The model under review builds one solid part; all positions refer to its coordinate system, in mm. A direction names the side the tool comes from. Coordinates: 2 decimals unless noted, no trailing zeros. Order: outer loops, then holes, each group sorted by start corner. A loop starts at its lowest first (then second) coordinate and runs counter-clockwise, first axis right, second up. Notation, with made-up numbers: M 64,45.25 L 112,45.25 A15 ccw 112,59.25 Z; hole C 59,42.5 d11. An arc over 180 degrees is marked long. Answer as CSV lines item,"result". Start each with the question number.
Q1. Consider section A-A on x = 10. Write out the cut boundary in (y, z), and give its area (4 significant figures).
Q2. Consider section D-D on y = 16. Write out the cut boundary in (x, z).
Q3. The part is to be moulded in two halves that separate along Y. For faces 4 (the face through (10, 15, 6.25)), 5 (the face through (0, 17.5, 5)), say which applies: +Y half, -Y half, draft (parallel to the pull), parting line (faces both ways), or undercut.
Q4. Consider section C-C on z = 1.75. Write out the cut boundary in (x, y).
Q5. Consider section B-B on z = 5.25. Write out the cut boundary in (x, y).
Q6. Machinability: for faces 1 (the face through (-10, 15, 6.25)), 2 (the face through (5, 15, 3)), 3 (the face through (0, 22.5, 5)), which of the approach directions +Z, -Z, +X, -X, +Y, -Y give a long, thin tool a straight path to every point of the face, cutting with its end or side? Answer none if there is none.
Q7. Wall thickness on L1, parallel to Y at x = 1.75, z = 7.5; L2, parallel to X at y = 3.5, z = 1.75; L3, parallel to X at y = 8.75, z = 7: over which ranges is each line inside the solid? List them lowest first. Write a range as [from, to].
Q8. For P1, Ø7, axis at x = 1, z = -1.5, coming from the +Y side; P2, Ø6.5, axis at x = 10, z = 1.75, coming from the +Y side; P3, Ø1, axis at x = -9.5, z = 3, coming from the +Y side; P4, Ø2.5, axis at x = 1, y = 19, coming from the +Z side, all flat-tipped, find the tip position at first contact; note any pin that passes through.
from build123d import *

# Parameters (mm, degrees)
SKETCH1_W           = 30
SKETCH1_H           = 16.5
SKETCH1_R           = 2.1
BOSS_EXTRUDE1_DEPTH = 5
SKETCH2_W           = 30
SKETCH2_H           = 20
BOSS_EXTRUDE2_DEPTH = 2
SKETCH3_W           = 5
SKETCH3_H           = 5
CUT_EXTRUDE1_DEPTH  = 3
SKETCH4_W           = 10
SKETCH4_H           = 20
SKETCH4_W_2         = 5
SKETCH4_H_2         = 5
BOSS_EXTRUDE3_DEPTH = 4
SKETCH5_W           = 10
SKETCH5_H           = 20
BOSS_EXTRUDE4_DEPTH = 2


with BuildPart() as part:
    # Sketch1 → Boss-Extrude1 (new body)
    with BuildSketch(Plane(origin=(0, 0, 0), x_dir=(1, 0, 0), z_dir=(0, 1, 0))):
        Rectangle(SKETCH1_W, SKETCH1_H)
        with Locations((-10, -1.75)):
            Circle(SKETCH1_R, mode=Mode.SUBTRACT)
        with Locations((10, -1.75)):
            Circle(SKETCH1_R, mode=Mode.SUBTRACT)
    extrude(amount=BOSS_EXTRUDE1_DEPTH)

    # Sketch2 → Boss-Extrude2 (add)
    with BuildSketch(Plane.XY.offset(8.25)):
        with Locations((0, 15)):
            Rectangle(SKETCH2_W, SKETCH2_H)
    extrude(amount=-BOSS_EXTRUDE2_DEPTH)

    # Sketch3 → Cut-Extrude1 (cut, through all)
    with BuildSketch(Plane(origin=(0, 0, 6.25), x_dir=(-1, 0, 0), z_dir=(0, 0, -1))):
        with Locations((0, 10)):
            Rectangle(SKETCH3_W, SKETCH3_H)
        with Locations((0, 20)):
            Rectangle(SKETCH3_W, SKETCH3_H)
    extrude(amount=-CUT_EXTRUDE1_DEPTH, mode=Mode.SUBTRACT)

    # Sketch4 → Boss-Extrude3 (add)
    with BuildSketch(Plane(origin=(0, 0, 6.25), x_dir=(-1, 0, 0), z_dir=(0, 0, -1))):
        with Locations((0, 15)):
            Rectangle(SKETCH4_W, SKETCH4_H)
        with Locations((0, 20)):
            Rectangle(SKETCH4_W_2, SKETCH4_H_2, mode=Mode.SUBTRACT)
        with Locations((0, 10)):
            Rectangle(SKETCH4_W_2, SKETCH4_H_2, mode=Mode.SUBTRACT)
    extrude(amount=BOSS_EXTRUDE3_DEPTH)

    # Sketch5 → Boss-Extrude4 (add)
    with BuildSketch(Plane(origin=(0, 0, 2.25), x_dir=(-1, 0, 0), z_dir=(0, 0, -1))):
        with Locations((0, 15)):
            Rectangle(SKETCH5_W, SKETCH5_H)
    extrude(amount=BOSS_EXTRUDE4_DEPTH)


solid = part.part
Evaluation:
1,outline,"M 0,-8.25 L 5,-8.25 L 5,-0.35 L 0,-0.35 Z; M 0,3.85 L 5,3.85 L 5,6.25 L 25,6.25 L 25,8.25 L 0,8.25 Z"
1,area,"101.5 mm²"
2,outline,"M -15,6.25 L -5,6.25 L -5,0.25 L 5,0.25 L 5,6.25 L 15,6.25 L 15,8.25 L -15,8.25 Z"
3,face 4,"draft"
3,face 5,"undercut"
4,outline,"M -15,0 L -12.1,0 L -12.1,5 L -15,5 Z; M -7.9,0 L 7.9,0 L 7.9,5 L 5,5 L 5,25 L -5,25 L -5,5 L -7.9,5 Z; M 12.1,0 L 15,0 L 15,5 L 12.1,5 Z"
5,outline,"M -15,0 L 15,0 L 15,5 L 5,5 L 5,25 L -5,25 L -5,5 L -15,5 Z; hole M -2.5,7.5 L 2.5,7.5 L 2.5,12.5 L -2.5,12.5 Z; hole M -2.5,17.5 L 2.5,17.5 L 2.5,22.5 L -2.5,22.5 Z"
6,face 1,"-Z, -X, +Y"
6,face 2,"-Z, +X, +Y"
6,face 3,"+Z"
7,L1,"y = [0, 7.5], [12.5, 17.5], [22.5, 25]"
7,L2,"x = [-15, -12.1], [-7.9, 7.9], [12.1, 15]"
7,L3,"x = [-15, -2.5], [2.5, 15]"
8,P1,"stops at y = 25"
8,P2,"stops at y = 5"
8,P3,"passes through"
8,P4,"stops at z = 2.25"
